Source: CAD feature listing. Evaluate the final solid. Frame: model axes, mm. A direction names the side the tool comes from. Give positions to 0.01 mm unless a question says otherwise; leave off trailing zeros. Order: outer loops, then holes, each group sorted by start corner. A loop starts at its lowest first (then second) coordinate and runs counter-clockwise, first axis right, second up. Notation, with made-up numbers: (68, 1.5) - (116, 1.5) arc R27 cw to (116, 38.5) - close; hole circle Ø4 at (59.25, 10.5). An arc over 180 degrees is marked (long way). Write each question's results on one line, items separated by ' | '. Start each with the question number.
Item 1: Section C-C on z = -5. Output: boundary loops of the cut face in (x, y).
Item 2: Section A-A on y = -4.5. State how many separate pieces and enclosed holes the cut face has, and give its area (3 significant figures).
Item 3: Contact query for flat-ended pins moving along their axis: pin 1 Ø3 at (x, y) = (24, -3.5) entering from -Z; pin 2 Ø1.5 at (x, y) = (2, 2) entering from +Z; pin 3 Ø5 at (y, z) = (-3, -15.5) entering from -X; pin 4 Ø1.5 at (x, z) = (-28, -20) entering from +Y. Output: stop coordinate, or through.
Item 4: Section B-B on x = -20.5. Output: boundary loops of the cut face in (y, z), and give its area (3 significant figures).
Item 5: Set-up query: faces 4 (the flat face through (-10, -1, -38.639)), 5 (the cylindrical face through (23.872, -2.89, -37.937)), 6 (the flat face through (-10, -2, -39.439)). Return all of +Z, -Z, +X, -X, +Y, -Y with unobstructed straight access to the full face (end or side cutting, diameter ignored); none if empty.
Item 6: Mould query, pull axis X, two halves, no side actions, for faces 1 (the flat face through (-10, 0, -40)), 2 (the flat face through (20.914, -3, 3)), 3 (the cylindrical face through (-49.285, 0.493, 12.79)). Classes: released by +X, released by -X, zero draft, split by the parting line, or undercut.
Item 7: Line query: line 1 along Z through (x, y) = (-46, -3.25); line 2 along X through (y, z) = (-1.75, -14); line 3 along Z through (x, y) = (-29, -1.5). Output: solid intervals per line, ascending.
```python
from build123d import *

# Parameters (mm, degrees)
SKETCH1_R           = 6.5
BOSS_EXTRUDE1_DEPTH = 3
FILLET1_R           = 2
SKETCH3_W           = 74
SKETCH3_H           = 50
SKETCH3_W_2         = 72
SKETCH3_H_2         = 48
BOSS_EXTRUDE2_DEPTH = 3
SKETCH4_W           = 74
SKETCH4_H           = 50
SKETCH4_W_2         = 73.6
SKETCH4_H_2         = 49.6
CUT_EXTRUDE1_DEPTH  = 3
FILLET2_R           = 1
SKETCH6_W           = 6
SKETCH6_H           = 8
BOSS_EXTRUDE3_DEPTH = 6
SKETCH7_R           = 2.5
CUT_EXTRUDE2_DEPTH  = 89.047516081


with BuildPart() as part:
    # Sketch1 → Boss-Extrude1 (new body)
    with BuildSketch(Plane(origin=(0, 0, 0), x_dir=(1, 0, 0), z_dir=(0, 1, 0))):
        with BuildLine():
            Line((-47.886115273, 42.639478046), (28.113884727, 42.639478046))
            ThreePointArc((28.113884727, 42.639478046), (29.528098289, 42.053691608), (30.113884727, 40.639478046))
            Line((30.113884727, 40.639478046), (30.113884727, -11.360521954))
            ThreePointArc((30.113884727, -11.360521954), (29.528098289, -12.774735517), (28.113884727, -13.360521954))
            Line((28.113884727, -13.360521954), (-47.886115273, -13.360521954))
            ThreePointArc((-47.886115273, -13.360521954), (-49.300328836, -12.774735517), (-49.886115273, -11.360521954))
            Line((-49.886115273, -11.360521954), (-49.886115273, 40.639478046))
            ThreePointArc((-49.886115273, 40.639478046), (-49.300328836, 42.053691608), (-47.886115273, 42.639478046))
        make_face()
        with Locations(Location((-29.886115273, 14.639478046, 0), (0, 0, 270))):
            Circle(SKETCH1_R, mode=Mode.SUBTRACT)
    extrude(amount=BOSS_EXTRUDE1_DEPTH)

    # Fillet1
    fillet1_edges = [part.edges().sort_by_distance(p)[0] for p in [
        (29.528098289, 3, -42.053691608),
        (-9.886115273, 3, -42.639478046),
        (-49.300328836, 3, -42.053691608),
        (-49.886115273, 3, -14.639478046),
        (-49.300328836, 3, 12.774735517),
        (-9.886115273, 3, 13.360521954),
        (29.528098289, 3, 12.774735517),
        (30.113884727, 3, -14.639478046),
    ]]
    fillet(fillet1_edges, radius=FILLET1_R)

    # Sketch3 → Boss-Extrude2 (add)
    with BuildSketch(Plane.XZ):
        with Locations((-9.886115273, -14.639478046)):
            Rectangle(SKETCH3_W, SKETCH3_H)
        with Locations((-9.886115273, -14.639478046)):
            Rectangle(SKETCH3_W_2, SKETCH3_H_2, mode=Mode.SUBTRACT)
    extrude(amount=BOSS_EXTRUDE2_DEPTH)

    # Sketch4 → Cut-Extrude1 (cut)
    with BuildSketch(Plane.XZ.offset(3)):
        with Locations((-9.886115273, -14.639478046)):
            Rectangle(SKETCH4_W, SKETCH4_H)
        with Locations((-9.886115273, -14.639478046)):
            Rectangle(SKETCH4_W_2, SKETCH4_H_2, mode=Mode.SUBTRACT)
    extrude(amount=-CUT_EXTRUDE1_DEPTH, mode=Mode.SUBTRACT)

    # Fillet2
    fillet2_edges = [part.edges().sort_by_distance(p)[0] for p in [
        (-29.886115273, 3, -21.139478046),
    ]]
    fillet(fillet2_edges, radius=FILLET2_R)

    # Sketch6 → Boss-Extrude3 (add)
    with BuildSketch(Plane.XZ):
        with Locations((-43.686115273, 6.160521954)):
            Rectangle(SKETCH6_W, SKETCH6_H)
        with Locations((23.913884727, 6.160521954)):
            Rectangle(SKETCH6_W, SKETCH6_H)
        with Locations((23.913884727, -35.439478046)):
            Rectangle(SKETCH6_W, SKETCH6_H)
        with Locations((-43.686115273, -35.439478046)):
            Rectangle(SKETCH6_W, SKETCH6_H)
    extrude(amount=BOSS_EXTRUDE3_DEPTH)

    # Sketch7 → Cut-Extrude2 (cut, through all)
    with BuildSketch(Plane.ZY.offset(46.686115273)):
        with Locations((-35.439478046, -3)):
            Circle(SKETCH7_R)
        with Locations(Location((6.160521954, -3, 0), (0, 0, 180))):
            Circle(SKETCH7_R)
    extrude(amount=-CUT_EXTRUDE2_DEPTH, mode=Mode.SUBTRACT)


solid = part.part
```
Evaluation:
1) outline: (-49.89, 0) - (-46.69, 0) - (-46.69, -3) - (-45.89, -3) - (-45.89, 0) - (26.11, 0) - (26.11, -3) - (26.91, -3) - (26.91, 0) - (30.11, 0) - (30.11, 1) arc R2 ccw to (28.11, 3) - (-47.89, 3) arc R2 ccw to (-49.89, 1) - close
2) separate pieces: 8 | enclosed holes: 0 | area: 96.0 mm^2
3) pin 1: stops at z = -39.44 | pin 2: stops at z = 13.34 | pin 3: stops at x = -46.69 | pin 4: passes through
4) outline: (-3, -39.44) - (0, -39.44) - (0, -42.64) - (1, -42.64) arc R2 ccw to (3, -40.64) - (3, 11.36) arc R2 ccw to (1, 13.36) - (0, 13.36) - (0, 10.16) - (-3, 10.16) - (-3, 9.36) - (0, 9.36) - (0, -38.64) - (-3, -38.64) - close | area: 171 mm^2
5) face 4: -Y | face 5: +X, -X | face 6: -Z, +X, -X, -Y
6) face 1: zero draft | face 2: undercut | face 3: released by -X
7) line 1: z = -39.44 to -37.93, -32.95 to -31.44, 2.16 to 3.67, 8.65 to 10.16 | line 2: x = -46.69 to -45.89, 26.11 to 26.91 | line 3: z = -39.44 to -38.64, 9.36 to 10.16
